Input: part model. Units: mm. Frame: model coordinates. Coordinates: 2 decimals unless noted, no trailing zeros. Order: outer loops, then holes, each group sorted by start corner. A loop starts at its lowest first (then second) coordinate and runs counter-clockwise, first axis right, second up. Notation, with made-up numbers: M 36.25,-13 L 83.25,-13 A28 cw 83.25,7 Z; hole C -6,75 d6. An arc over 180 degrees is marked long. Answer in a Markdown table with one row per item.
Autodesk Fusion 360 part; units mm, degrees
sketch "Sketch1" plane through (0, 0, 0) normal (0, 1, 0) x (1, 0, 0)
  circle A0 centre (0, 0) radius 9.5
  circle A1 centre (0, 0) radius 2.1
  circle A2 centre (6, 0) radius 1.25
  circle A3 centre (0, 0) radius 6 construction
  circle A4 centre (0, 6) radius 1.25
  circle A5 centre (-6, 0) radius 1.25
  circle A6 centre (0, -6) radius 1.25
  dimension "d1" = 19
  dimension "d2" = 4.2
  dimension "d3" = 2.5
  dimension "d5" = 360
extrude "Extrude1" add sketch "Sketch1" along normal blind 5.1
chamfer "Chamfer1" distance 0.3 angle 45 2 edges at (-8.8571, 5.1, 3.4353) (-8.8571, 0, 3.4353)
chamfer "Chamfer2" distance 0.3 angle 45 10 edges at (-1.9579, 5.1, -0.7594) (-1.1654, 5.1, -6.452) (-7.1654, 5.1, -0.452) (-1.1654, 5.1, 5.548) (4.8346, 5.1, -0.452) (-1.1654, 0, 5.548) (-7.1654, 0, -0.452) (-1.1654, 0, -6.452) (-1.9579, 0, -0.7594) (4.8346, 0, -0.452)
1) Mould query, pull axis X, two halves, no side actions, for faces 1 (the face through (4.38, 2.52, -8.43)), 2 (the face through (2, 0, 2)), 3 (the face through (-0.27, 2.52, 4.78)). Classes: +X half, -X half, draft (parallel to the pull), parting line (faces both ways), or undercut.
Resolved:
| item | result |
|---|---|
| face 1 | parting line |
| face 2 | draft |
| face 3 | undercut |
2) Contact query for flat-ended pins moving along their axis: pin 1 (1.5 mm diameter, centred on x = -0.5, z = 2, fed in from -Y); pin 2 (3 mm diameter, centred on x = 0, z = -6, fed in from +Y); pin 3 (3 mm diameter, centred on y = 2.5, z = -3, fed in from -X). Output: stop coordinate, or through.
Resolved:
| item | result |
|---|---|
| pin 1 | stops at y = 0 |
| pin 2 | stops at y = 5.05 |
| pin 3 | stops at x = -9.38 |
3) Cut plane C-C, the plane y = 1.35. Output: boundary loops of the cut face in (x, z).
Resolved:
| item | result |
|---|---|
| outline | C 0,0 d19; hole C -6,0 d2.5; hole C 0,0 d4.2; hole C 0,-6 d2.5; hole C 0,6 d2.5; hole C 6,0 d2.5 |
4) Cut plane A-A, the plane z = 0. State how many separate pieces and enclosed holes the cut face has, and give its area (3 significant figures).
Resolved:
| item | result |
|---|---|
| separate pieces | 4 |
| enclosed holes | 0 |
| area | 49.3 mm2 |
5) Material intervals for probe 1 along X at (y, z) = (2.9, 0); probe 2 along Z at (x, y) = (5.5, 4.15), sorted ascending.
Resolved:
| item | result |
|---|---|
| probe 1 | x = -9.5 to -7.25, -4.75 to -2.1, 2.1 to 4.75, 7.25 to 9.5 |
| probe 2 | z = -7.75 to -1.15, 1.15 to 7.75 |
